The model under review builds one solid part; all positions refer to its coordinate system, in mm. A direction names the side the tool comes from. Round coordinates to 2 decimals unless told otherwise and drop trailing zeros. Write each loop counter-clockwise with the first axis right and the second up, starting at its lowest first coordinate (ties: lowest second). Pieces come first, ordered by that corner, then holes. Notation, with made-up numbers: (8.25, -24.75) -> (48.25, -24.75) arc R29 cw to (48.25, -4.75) -> close; hole circle Ø1 at (54, -7). An arc over 180 degrees is marked (long way). Return JSON: item names as keys, results as strings. Group by question number.
1. Take a section at C-C, the plane y = 2.5. Write out the cut boundary in (x, z), then the cut area to 3 significant figures.
2. Tool access review of faces 4 (the flat face through (-0.829, 4, 0)), 5 (the cylindrical face through (1.73, 1.48, 7.81)), 6 (the cylindrical face through (1.08, 8.96, 4.88)): name each direction out of +Z, -Z, +X, -X, +Y, -Y from which nothing blocks a thin tool from reaching the whole face with its end or side.
3. Take a section at D-D, the plane y = 10.25. Write out the cut boundary in (x, z), then the cut area to 3 significant figures.
4. Mouldability with a two-part tool opening along Z and no side actions: class faces 1 (the cylindrical face through (1.73, 16.48, 7.81)), 2 (the flat face through (0, 8, 0)), 3 (the flat face through (0, 0, -2)) as pulls with the +Z half, pulls with the -Z half, needs draft (parallel to the pull), parting line crosses it, or undercut.
5. Clearance check with flat-ended pins moving along their axes: P1, Ø1.2, axis at x = 0.5, z = 0, coming from the -Y side; P2, Ø1, axis at x = -6, y = 3, coming from the +Z side; P3, Ø1.5, axis at y = 11, z = -6, coming from the -X side; P4, Ø1, axis at x = -2, y = 4.5, coming from the -Z side. State where each tip first meets the part, or that it passes through.
6. For line 1 along Z through (x, y) = (0, 2.5); line 2 along Y through (x, z) = (-6, -2); line 3 along Y through (x, z) = (-7, 1), list the stretches that pass through material, from the lowest coordinate up. Write a range as from..to.
Autodesk Inventor part; units mm, degrees
ref_plane "YZ Plane" through (0, 0, 0) normal (1, 0, 0) x (0, 1, 0)
ref_plane "XZ Plane" through (0, 0, 0) normal (0, 1, 0) x (-1, 0, 0)
ref_plane "XY Plane" through (0, 0, 0) normal (0, 0, 1) x (1, 0, 0)
sketch "Szkic1" plane through (0, 0, 0) normal (0, 1, 0) x (-1, 0, 0)
  circle A0 centre (0, 0) radius 8
  circle A1 centre (0, 0) radius 5
  arc A2 (0.8292, 1.25) -> (0.8292, -1.25) centre (0, 0) ccw
  line L0 (0.8292, 1.25) -> (0.8292, -1.25)
  dimension "d2" = 1.5
  dimension "d3" = 2.5
  dimension "d4" = 10
  dimension "d5" = 16
extrude "Wyciągnięcie proste1" add sketch "Szkic1" along normal blind 18 contours A0 | A1 | L0 A2
extrude "Wyciągnięcie proste2" cut sketch "Szkic1" along normal blind 15 contours A0
extrude "Wyciągnięcie proste3" add sketch "Szkic1" along normal blind 3 contours A0
extrude "Wyciągnięcie proste4" cut sketch "Szkic1" along normal blind 8 contours L0 A2
chamfer "Faza1" distance 3 angle 45 2 edges at (5, 3, 0) (5, 15, 0)
properties part number "kolo_napedowe" material "PLA"
Output:
{
 "1": {"outline": "circle Ø16 at (0, 0); hole (-0.83, -1.25) arc R1.5 ccw (long way) to (-0.83, 1.25) -> close", "area": "195 mm^2"},
 "2": {"face 4": "-Y", "face 5": "+Y, -Y", "face 6": "none"},
 "3": {"outline": "circle Ø10 at (0, 0)", "area": "78.5 mm^2"},
 "4": {"face 1": "parting line crosses it", "face 2": "undercut", "face 3": "needs draft"},
 "5": {"P1": "stops at y = 8", "P2": "stops at z = 5.81", "P3": "passes through", "P4": "stops at z = -6.73"},
 "6": {"line 1": "z = -8..-1.5, 1.5..8", "line 2": "y = 0..4.67, 13.33..18", "line 3": "y = 0..3.93, 14.07..18"}
}
